from build123d import *

# Parameters (mm, degrees)
F0_W     = 57.15
F0_H     = 38.1
F1_DEPTH = 25.4
F3_DEPTH = 25.4
F5_DEPTH = 25.4


with BuildPart() as f1:
    # F0 (on Front) → F1 (new body)
    with BuildSketch(Plane.XZ):
        with Locations((28.575, 19.05)):
            Rectangle(F0_W, F0_H)
    extrude(amount=F1_DEPTH)

    # F2 (on face) → F3 (cut)
    with BuildSketch(Plane.XZ.offset(25.4)):
        with BuildLine():
            Line((57.15, 38.1), (38.1, 38.1))
            ThreePointArc((38.1, 38.1), (43.167062, 24.117062), (57.15, 19.05))
            Line((57.15, 19.05), (57.15, 38.1))
        make_face()
    extrude(amount=-F3_DEPTH, mode=Mode.SUBTRACT)

    # F4 (on face) → F5 (cut)
    with BuildSketch(Plane.XZ.offset(25.4)):
        with BuildLine():
            ThreePointArc((0, 31.75), (2.621624, 35.478376), (6.35, 38.1))
            Line((6.35, 38.1), (0, 38.1))
            Line((0, 38.1), (0, 31.75))
        make_face()
    extrude(amount=-F5_DEPTH, mode=Mode.SUBTRACT)


solid = f1.part
Geometry: final body of the model. Coordinates: model frame, mm. Give positions to 0.01 mm unless a question says otherwise; leave off trailing zeros. Order: outer loops, then holes, each group sorted by start corner. A loop starts at its lowest first (then second) coordinate and runs counter-clockwise, first axis right, second up. Notation, with made-up numbers: (-15.5, 17) -> (35.5, 17) arc R19 cw to (35.5, 42) -> close; hole circle Ø6 at (26.25, 62). An arc over 180 degrees is marked (long way). Write each question's results on one line, items separated by ' | '.
1) Line query: line 1 along Z through (x, y) = (53, -15.25); line 2 along X through (y, z) = (-13.5, 35) (3 decimals); line 3 along Z through (x, y) = (52.5, -12.5). Output: solid intervals per line, ascending.
Geometry says:
line 1: z = 0 to 19.17 | line 2: x = 2.166 to 38.095 | line 3: z = 0 to 19.25
2) Cut plane A-A (y = -2). Output: boundary loops of the cut face in (x, z).
Geometry says:
outline: (0, 0) -> (57.15, 0) -> (57.15, 19.05) arc R17.54 cw to (38.1, 38.1) -> (6.35, 38.1) arc R13.27 ccw to (0, 31.75) -> close
3) Cut plane C-C (x = 47). Output: boundary loops of the cut face in (y, z).
Geometry says:
outline: (-25.4, 0) -> (0, 0) -> (0, 21.22) -> (-25.4, 21.22) -> close
4) Cut plane B-B (z = 25). Output: boundary loops of the cut face in (x, y), and give its area (3 significant figures).
Geometry says:
outline: (0, -25.4) -> (42.34, -25.4) -> (42.34, 0) -> (0, 0) -> close | area: 1,080 mm²
